Model file for the job. Use its own axes, mm. Round coordinates to 2 decimals unless told otherwise and drop trailing zeros. Order: outer loops, then holes, each group sorted by start corner. A loop starts at its lowest first (then second) coordinate and runs counter-clockwise, first axis right, second up. Notation, with made-up numbers: (75, 37) - (96, 37) arc R14 cw to (96, 56) - close; hole circle Ø3 at (5.25, 86.25). An arc over 180 degrees is marked (long way). Answer as CSV lines item,"result". Start each with the question number.
1. Band-saw the part on A-A on z = -5. List the corners of the cut face in (x, y) (3 decimals).
2. Wall check: line 1 along Z through (x, y) = (15, -1.75); line 2 along Z through (x, y) = (23.75, -2.5); line 3 along X through (y, z) = (-2.4, -14.5). Give the ranges that are in metal, low to high. Write a range as [from, to].
3. Pull direction Z, two halves, no side cores. Call faces 1 (the face through (29.236, -1.565, -29.276)), 2 (the face through (4.792, -1.565, -23.414)), 3 (the face through (15, -2, 0)), 4 (the face through (30, -2, -15)): released by +Z, released by -Z, zero draft, split by the parting line, or undercut.
4. Band-saw the part on C-C on x = 25. List the corners of the cut face in (y, z) (3 decimals).
5. Band-saw the part on B-B on y = -0.95. State how many separate pieces and enclosed holes the cut face has, then the cut area to 3 significant figures.
```python
from build123d import *

# Parameters (mm, degrees)
F0_R     = 1.6
F1_DEPTH = 3.175


# Not quite as in the source:
# - a length typed as a fraction of an inch, garbled in the dataset ("3 / 203.2 mm" for 3/8 in), is restored


with BuildPart() as f1:
    # F0 (on Front) → F1 (new body)
    with BuildSketch(Plane.XZ):
        with BuildLine():
            Line((27.46, 0), (2.54, 0))
            ThreePointArc((2.54, 0), (0.7439487758, -0.7439487758), (0, -2.54))
            Line((0, -2.54), (0, -27.46))
            ThreePointArc((0, -27.46), (0.7439487758, -29.2560512242), (2.54, -30))
            Line((2.54, -30), (27.46, -30))
            ThreePointArc((27.46, -30), (29.2560512242, -29.2560512242), (30, -27.46))
            Line((30, -27.46), (30, -2.54))
            ThreePointArc((30, -2.54), (29.2560512242, -0.7439487758), (27.46, 0))
        make_face()
        with Locations((5, -25)):
            Circle(F0_R, mode=Mode.SUBTRACT)
        with Locations((15, -25)):
            Circle(F0_R, mode=Mode.SUBTRACT)
        with Locations((25, -25)):
            Circle(F0_R, mode=Mode.SUBTRACT)
        with Locations((5, -15)):
            Circle(F0_R, mode=Mode.SUBTRACT)
        with Locations((5, -5)):
            Circle(F0_R, mode=Mode.SUBTRACT)
        with Locations((15, -15)):
            Circle(F0_R, mode=Mode.SUBTRACT)
        with Locations((25, -15)):
            Circle(F0_R, mode=Mode.SUBTRACT)
        with Locations((15, -5)):
            Circle(F0_R, mode=Mode.SUBTRACT)
        with Locations((25, -5)):
            Circle(F0_R, mode=Mode.SUBTRACT)
    extrude(amount=F1_DEPTH)


solid = f1.part
```
Reply:
1,outline,"(0, -3.175) - (3.4, -3.175) - (3.4, 0) - (0, 0) - close; (6.6, -3.175) - (13.4, -3.175) - (13.4, 0) - (6.6, 0) - close; (16.6, -3.175) - (23.4, -3.175) - (23.4, 0) - (16.6, 0) - close; (26.6, -3.175) - (30, -3.175) - (30, 0) - (26.6, 0) - close"
2,line 1,"z = [-30, -26.6], [-23.4, -16.6], [-13.4, -6.6], [-3.4, 0]"
2,line 2,"z = [-30, -26], [-24, -16], [-14, -6], [-4, 0]"
2,line 3,"x = [0, 3.48], [6.52, 13.48], [16.52, 23.48], [26.52, 30]"
3,face 1,"released by -Z"
3,face 2,"undercut"
3,face 3,"released by +Z"
3,face 4,"zero draft"
4,outline,"(-3.175, -30) - (0, -30) - (0, -26.6) - (-3.175, -26.6) - close; (-3.175, -23.4) - (0, -23.4) - (0, -16.6) - (-3.175, -16.6) - close; (-3.175, -13.4) - (0, -13.4) - (0, -6.6) - (-3.175, -6.6) - close; (-3.175, -3.4) - (0, -3.4) - (0, 0) - (-3.175, 0) - close"
5,separate pieces,"1"
5,enclosed holes,"9"
5,area,"822 mm2"
